Part model, mm, in its own coordinate system. Face numbers are marked on the shaded views. Coordinates: 2 decimals unless noted, no trailing zeros. Write each loop counter-clockwise with the first axis right and the second up, starting at its lowest first coordinate (ties: lowest second). Pieces come first, ordered by that corner, then holes. Notation, with made-up numbers: M 79.5,3 L 94.5,3 A12 cw 94.5,18 Z; hole C 30.25,-13.5 d2. An arc over 180 degrees is marked long. Use a Markdown table: item, result. Add a question column.
Q1. Slice it at C-C on y = -56. Write the cut outline in (x, z), then the cut area to 3 significant figures.
Q2. Slice it at B-B on x = 5. Write the cut outline in (y, z), then the cut area to 3 significant figures.
Q3. Mould opens along X. For the marked faces 1, 2 and 3 say: released by +X, released by -X, zero draft, split by the parting line, or undercut.
Q4. Slice it at A-A on y = 0. Count the separate pieces of the cut face and the enclosed holes in it, then the cut area to 3 significant figures.
Q5. Pin check, flat tips, straight feed: pin 1 Ø6 at (x, z) = (-27.5, 3.5) entering from +Y; pin 2 Ø4 at (y, z) = (-30, 3) entering from +X; pin 3 Ø5 at (y, z) = (18.5, 3) entering from +X. Stop position of each tip, or through.
Q6. Wall check: L1, parallel to X at y = -19, z = 9.5; L2, parallel to X at y = 52.5, z = 1.5; L3, parallel to Y at x = 52, z = 1. Give the ranges that are in metal, low to high. Write a range as from..to.
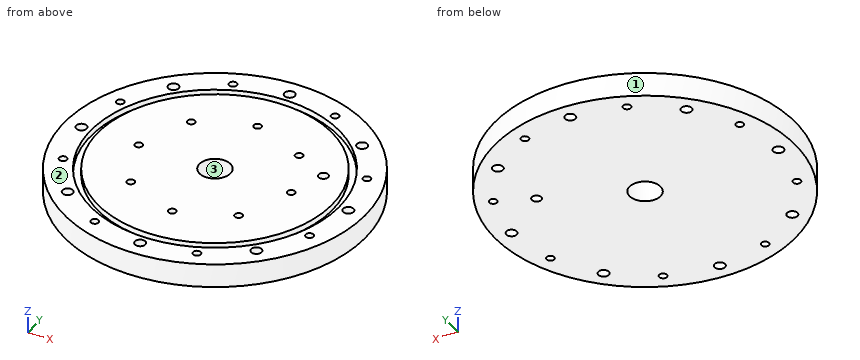
Autodesk Inventor part; units mm, degrees
ref_plane "YZ Plane" through (0, 0, 0) normal (1, 0, 0) x (0, 1, 0)
ref_plane "XZ Plane" through (0, 0, 0) normal (0, 1, 0) x (-1, 0, 0)
ref_plane "XY Plane" through (0, 0, 0) normal (0, 0, 1) x (1, 0, 0)
sketch "Sketch1" plane through (0, 0, 0) normal (0, 0, 1) x (1, 0, 0)
  circle A0 centre (0, 0) radius 63
  dimension "d0" = 126
extrude "Extrusion1" add sketch "Sketch1" along normal blind 10
sketch "Sketch3" plane through (0, 0, 10) normal (0, 0, 1) x (1, 0, 0)
  circle A0 centre (0, 0) radius 52
  circle A1 centre (0, 0) radius 49
  dimension "d11" = 3
  dimension "d35" = 98
extrude "Extrusion3" cut sketch "Sketch3" against normal blind 2.5
sketch "Sketch2" plane through (0, 0, 10) normal (0, 0, 1) x (1, 0, 0)
  circle A0 centre (0, 0) radius 56 construction
  circle A1 centre (0, 56) radius 2.2
  line L0 (0, -88.2) -> (0, 88.2)
  dimension "d3" = 112
  dimension "d4" = 4.4
extrude "Extrusion2" cut sketch "Sketch2" against normal blind 10
pattern_circular "Circular Pattern1" count 8 over 360 about axis through (0, 0, -10) along (0, 0, 1) of "Extrusion2"
sketch "Sketch4" plane through (0, 0, 10) normal (0, 0, 1) x (1, 0, 0)
  circle A0 centre (0, 0) radius 32 construction
  line L0 (0, -88.2) -> (0, 88.2) construction
  point P0 (0, 32)
  dimension "d14" = 64
hole "Hole1" at (0, 32, 10) direction (0, 0, -1) diameter 3.242 depth 8
pattern_circular "Circular Pattern2" count 8 over 360 about axis through (0, 0, -10) along (0, 0, 1) of "Hole1"
sketch "Sketch5" plane through (0, 0, 10) normal (0, 0, 1) x (1, 0, 0)
  circle A0 centre (36.9552, 15.3073) radius 2
  circle A1 centre (22.6274, 22.6274) radius 1.621 construction
  line L0 (22.6274, 22.6274) -> (0, 0) construction
  line L1 (0, 0) -> (36.9552, 15.3073) construction
  line L2 (-88.2, 0) -> (88.2, 0) construction
  circle A2 centre (0, 0) radius 42 construction
  dimension "d25" = 4
  dimension "d26" = 45
  dimension "d27" = 22.5
  dimension "d29" = 84
extrude "Extrusion4" cut sketch "Sketch5" against normal through all
sketch "Sketch6" plane through (0, 0, 10) normal (0, 0, 1) x (1, 0, 0)
  circle A0 centre (0, 0) radius 6.5
  dimension "d32" = 13
extrude "Extrusion5" cut sketch "Sketch6" against normal through all
sketch "Sketch7" plane through (0, 0, 10) normal (0, 0, 1) x (1, 0, 0)
  circle A0 centre (0, 56) radius 2.2 construction
  circle A1 centre (0, 0) radius 56 construction
  line L0 (-21.4303, 51.7373) -> (0, 0) construction
  line L1 (0, 0) -> (0, 56) construction
  circle A2 centre (-39.598, 39.598) radius 2.2 construction
  line L2 (-39.598, 39.598) -> (0, 0) construction
  dimension "d36" = 45
  dimension "d37" = 22.5
hole "Hole2" at (-21.4303, 51.7373, 10) direction (0, 0, -1) diameter 3.242 end through all
pattern_circular "Circular Pattern3" count 8 over 360 about axis through (0, 0, -10) along (0, 0, 1) of "Hole2"
equation "\"d27\" = 0.5 * d26"
equation "\"d37\" = 0.5 * d36"
properties part number "Base_Bowl_Glovebox" material "Aluminum 6061"
Recorded:
| question | item | result |
|---|---|---|
| 1 | outline | M -28.86,0 L -2.2,0 L -2.2,10 L -28.86,10 Z; M 2.2,0 L 28.86,0 L 28.86,10 L 2.2,10 Z |
| 1 | area | 533 mm² |
| 2 | outline | M -62.8,0 L -4.15,0 L -4.15,10 L -48.74,10 L -48.74,7.5 L -51.76,7.5 L -51.76,10 L -62.8,10 Z; M 4.15,0 L 62.8,0 L 62.8,10 L 51.76,10 L 51.76,7.5 L 48.74,7.5 L 48.74,10 L 4.15,10 Z |
| 2 | area | 1,160 mm² |
| 3 | face 1 | split by the parting line |
| 3 | face 2 | zero draft |
| 3 | face 3 | undercut |
| 4 | separate pieces | 4 |
| 4 | enclosed holes | 0 |
| 4 | area | 975 mm² |
| 5 | pin 1 | y = 58.04 |
| 5 | pin 2 | x = 56.44 |
| 5 | pin 3 | x = 60.93 |
| 6 | L1 | -60.07..-48.4, -45.17..45.17, 48.4..60.07 |
| 6 | L2 | -34.82..-22.86, -20..20, 22.86..34.82 |
| 6 | L3 | -35.57..-23.03, -19.83..19.83, 23.03..35.57 |
